Read the model definition and answer for the solid it produces. Units are mm, in the model's axes. Face numbers are marked on the shaded views. A direction names the side the tool comes from. Round coordinates to 2 decimals unless told otherwise and drop trailing zeros. Loops run counter-clockwise (first coordinate to the right, second up) from the corner with the lowest first, then second, coordinate; pieces in that order, holes last. Notation, with made-up numbers: (78, -26.5) - (91, -26.5) arc R28 cw to (91, 6.5) - close; hole circle Ø2 at (-20, 86.25). An arc over 180 degrees is marked (long way). Use one line per item in the form item = value. Start each with the question number.
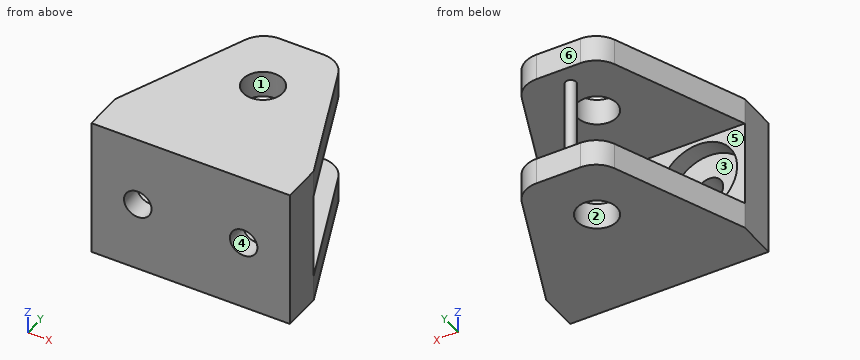
```python
from build123d import *

# Parameters (mm, degrees)
SKETCH1_W                               = 47.625
SKETCH1_H                               = 33.3502
BOSS_EXTRUDE1_DEPTH                     = 44.45
SKETCH2_W                               = 47.625
SKETCH2_H                               = 20.6502
CUT_EXTRUDE1_DEPTH                      = 34.925
CUT_EXTRUDE2_DEPTH                      = 61.457203841
CUT_EXTRUDE2_DEPTH_BACK                 = 61.457203841
CBORE_FOR_M6_HEX_HEAD_BOLT1_D           = 6.6
CBORE_FOR_M6_HEX_HEAD_BOLT1_DEPTH       = 14.019159957
CBORE_FOR_M6_HEX_HEAD_BOLT1_CBORE_D     = 18.55
CBORE_FOR_M6_HEX_HEAD_BOLT1_CBORE_DEPTH = 4.38
CBORE_FOR_M6_HEX_HEAD_BOLT1_TIP         = 1.982840043
FILLET3_R                               = 6.35
F_3_8_0_375_DIAMETER_HOLE1_D            = 9.525
BOSS_EXTRUDE2_REACH                     = 59.2
SKETCH15_R                              = 1.27


with BuildPart() as part:
    # Sketch1 → Boss-Extrude1 (new body)
    with BuildSketch(Plane(origin=(0, 0, 0), x_dir=(1, 0, 0), z_dir=(0, 1, 0))):
        Rectangle(SKETCH1_W, SKETCH1_H)
    extrude(amount=BOSS_EXTRUDE1_DEPTH)

    # Sketch2 → Cut-Extrude1 (cut)
    with BuildSketch(Plane(origin=(0, 44.45, 0), x_dir=(1, 0, 0), z_dir=(0, 1, 0))):
        Rectangle(SKETCH2_W, SKETCH2_H)
    extrude(amount=-CUT_EXTRUDE1_DEPTH, mode=Mode.SUBTRACT)

    # Sketch3 → Cut-Extrude2 (cut, two sides: drawn at the far end of the back side and taken through both)
    with BuildSketch(Plane(origin=(0, 0, -16.6751), x_dir=(-1, 0, 0), z_dir=(0, 0, -1)).offset(-CUT_EXTRUDE2_DEPTH_BACK)):
        Polygon((23.8125, 44.45), (9.525, 44.45), (23.8125, 9.525), align=None)
        Polygon((-23.8125, 9.525), (-9.525, 44.45), (-23.8125, 44.45), align=None)
    extrude(amount=CUT_EXTRUDE2_DEPTH + CUT_EXTRUDE2_DEPTH_BACK, mode=Mode.SUBTRACT)

    # CBORE for M6 Hex Head Bolt1
    with Locations(Plane(origin=(0, 9.525, 0), x_dir=(1, 0, 0), z_dir=(0, 1, 0))):
        with Locations((-12.7, 0), (12.7, 0)):
            CounterBoreHole(CBORE_FOR_M6_HEX_HEAD_BOLT1_D / 2, CBORE_FOR_M6_HEX_HEAD_BOLT1_CBORE_D / 2, CBORE_FOR_M6_HEX_HEAD_BOLT1_CBORE_DEPTH, depth=CBORE_FOR_M6_HEX_HEAD_BOLT1_DEPTH)
            with Locations((0, 0, -(CBORE_FOR_M6_HEX_HEAD_BOLT1_DEPTH + CBORE_FOR_M6_HEX_HEAD_BOLT1_TIP / 2))):  # 118° drill point
                Cone(0, CBORE_FOR_M6_HEX_HEAD_BOLT1_D / 2, CBORE_FOR_M6_HEX_HEAD_BOLT1_TIP, mode=Mode.SUBTRACT)

    # Fillet3
    fillet3_edges = [part.edges().sort_by_distance(p)[0] for p in [
        (9.525, 44.45, 13.5001),
        (-9.525, 44.45, 13.5001),
        (9.525, 44.45, -13.5001),
        (-9.525, 44.45, -13.5001),
    ]]
    fillet(fillet3_edges, radius=FILLET3_R)

    # 3/8 (0.375) Diameter Hole1 (through all)
    with Locations(Plane.XY.offset(16.6751)):
        with Locations((0, 28.969467427)):
            Hole(F_3_8_0_375_DIAMETER_HOLE1_D / 2)

    # Sketch15 → Boss-Extrude2 (add, up to next)
    with BuildSketch(Plane.XY.offset(-10.3251), mode=Mode.PRIVATE) as boss_extrude2_sk1:
        with Locations(Location((0, 39.468275157, 0), (0, 0, 180))):
            Circle(SKETCH15_R)
    boss_extrude2_tool1 = extrude(boss_extrude2_sk1.sketch, amount=BOSS_EXTRUDE2_REACH, mode=Mode.PRIVATE) - part.part
    add(boss_extrude2_tool1.solids().sort_by_distance((0, 39.468275, -10.3251))[0])


solid = part.part
```
1) A cutting plane is placed at B-B on z = -4. Write down the section's boundary in (x, y) (1 decimal), plus the area to 3 significant figures.
2) A cutting plane is placed at C-C on y = 35.5. Write down the section's boundary in (x, z), plus the area to 3 significant figures.
3) Determine the mould class of the marked faces 1, 2, 3 and 4 for opening direction Y: +Y half, -Y half, draft (parallel to the pull), parting line (faces both ways), or undercut.
4) A cutting plane is placed at A-A on x = 0. Write down the section's boundary in (y, z) (3 decimals).
5) Straight lines are drawn through the part: line 1 (Z direction, x = -12.7, y = 6.45) (3 decimals); line 2 (Z direction, x = -11.5, y = 12); line 3 (Y direction, x = -7, z = 5.5) (3 decimals). For each, find the intervals that lie inside material, in ascending order. Write a range as from..to.
6) A cutting plane is placed at D-D on z = 2.5. Write down the section's boundary in (x, y) (1 decimal), plus the area to 3 significant figures.
7) For the marked faces 5 and 6, determine the directions among +Z, -Z, +X, -X, +Y, -Y from which every point of the face is accessible in a straight line to the end or side of a thin tool.
8) Flat-ended cylindrical pins translate along their axes: pin 1 (5.5 mm diameter, centred on x = -15, z = 4, fed in from +Y) (3 decimals); pin 2 (2 mm diameter, centred on y = 40, z = -12, fed in from -X); pin 3 (1 mm diameter, centred on y = 38, z = -11.5, fed in from -X). Find the tip coordinate at first contact, or state that the pin passes through.
Checks:
q1.outline = (-23.8, 0) - (23.8, 0) - (23.8, 9.5) - (21.1, 9.5) - (21.1, 5.1) - (4.3, 5.1) - (4.3, 9.5) - (-4.3, 9.5) - (-4.3, 5.1) - (-21.1, 5.1) - (-21.1, 9.5) - (-23.8, 9.5) - close; circle Ø2.5 at (0, 39.5)
q1.area = 312 mm²
q2.outline = (-13.19, -16.68) - (13.19, -16.68) - (13.19, -10.33) - (-13.19, -10.33) - close; (-13.19, 10.33) - (13.19, 10.33) - (13.19, 16.68) - (-13.19, 16.68) - close
q2.area = 335 mm²
q3.face_1 = undercut
q3.face_2 = undercut
q3.face_3 = +Y half
q3.face_4 = draft
q4.outline = (0, -16.675) - (24.207, -16.675) - (24.207, -10.325) - (9.525, -10.325) - (9.525, 10.325) - (24.207, 10.325) - (24.207, 16.675) - (0, 16.675) - close; (33.732, -16.675) - (44.45, -16.675) - (44.45, -10.325) - (40.738, -10.325) - (40.738, 10.325) - (44.45, 10.325) - (44.45, 16.675) - (33.732, 16.675) - (33.732, 10.325) - (38.198, 10.325) - (38.198, -10.325) - (33.732, -10.325) - close
q5.line_1 = -16.675..-9.275, 9.275..16.675
q5.line_2 = -16.68..-10.33, 10.33..16.68
q5.line_3 = 0..5.145
q6.outline = (-23.8, 0) - (-14.9, 0) - (-14.9, 5.1) - (-21.6, 5.1) - (-21.6, 9.5) - (-23.8, 9.5) - close; (-10.5, 0) - (10.5, 0) - (10.5, 5.1) - (3.8, 5.1) - (3.8, 9.5) - (-3.8, 9.5) - (-3.8, 5.1) - (-10.5, 5.1) - close; circle Ø2.5 at (0, 39.5); (14.9, 0) - (23.8, 0) - (23.8, 9.5) - (21.6, 9.5) - (21.6, 5.1) - (14.9, 5.1) - close
q6.area = 258 mm²
q7.face_5 = +X, -X
q7.face_6 = +Z, -Z, +X, -X, +Y
q8.pin_1 = 5.145
q8.pin_2 = -11.75
q8.pin_3 = -12.37
